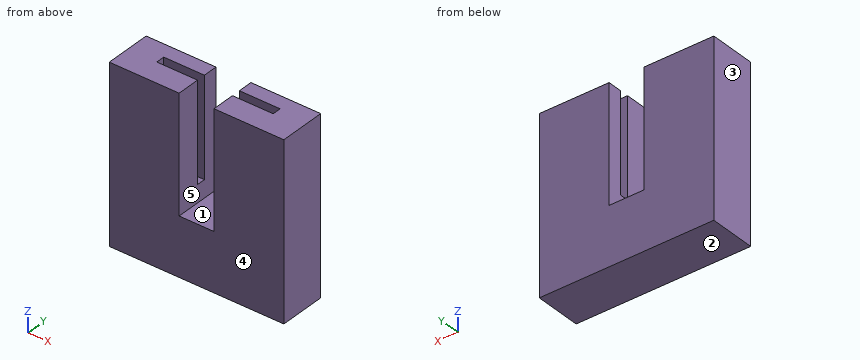
```python
from build123d import *

# Parameters (mm, degrees)
F0_W     = 30
F0_H     = 8
F1_DEPTH = 30
F3_W     = 6
F3_H     = 2.5
F3_H_2   = 4
F4_DEPTH = 20
F2_W     = 20
F2_H     = 1.5
F5_DEPTH = 20
F6_W     = 7
F6_H     = 1.5
F7_DEPTH = 3


with BuildPart() as f1:
    # F0 (on Top) → F1 (new body)
    with BuildSketch(Plane.XY):
        with Locations((-15, -4)):
            Rectangle(F0_W, F0_H)
    extrude(amount=F1_DEPTH)

    # F3 (on face) → F4 (cut)
    with BuildSketch(Plane.XY.offset(30)):
        with Locations((-15, -1.25)):
            Rectangle(F3_W, F3_H)
        with Locations((-15, -6)):
            Rectangle(F3_W, F3_H_2)
    extrude(amount=-F4_DEPTH, mode=Mode.SUBTRACT)

    # F2 (on face) → F5 (cut)
    with BuildSketch(Plane.XY.offset(30)):
        with Locations((-15, -3.25)):
            Rectangle(F2_W, F2_H)
    extrude(amount=-F5_DEPTH, mode=Mode.SUBTRACT)

    # F6 (on face) → F7 (join)
    with BuildSketch(Plane.XY.offset(10)):
        with Locations((-8.5, -3.25)):
            Rectangle(F6_W, F6_H)
        with Locations((-21.5, -3.25)):
            Rectangle(F6_W, F6_H)
    extrude(amount=F7_DEPTH)


solid = f1.part
```
For this review, take the finished solid that the model builds, in its own axes (mm). Face numbers are marked on the shaded views. A direction names the side the tool comes from. Coordinates: 2 decimals unless noted, no trailing zeros. Loops run counter-clockwise (first coordinate to the right, second up) from the corner with the lowest first, then second, coordinate; pieces in that order, holes last.
1. Add section B-B, the plane y = -5.25. Give the boundary of the cut face in (x, z), then the cut area to 3 significant figures.
2. Add section D-D, the plane z = 23.5. Give the boundary of the cut face in (x, y), then the cut area to 3 significant figures.
3. For the marked faces 4 and 5, list the 3-axis set-ups (+Z, -Z, +X, -X, +Y, -Y) from which the entire face can be reached by the end or side of a thin tool; tool diameter is ignored.
4. Add section C-C, the plane x = -8.25. Give the boundary of the cut face in (y, z).
5. Add section A-A, the plane z = 12.5. Give the boundary of the cut face in (x, y).
6. Mouldability with a two-part tool opening along X and no side actions: class the marked faces 1, 2 and 3 as +X half, -X half, draft (parallel to the pull), parting line (faces both ways), or undercut.
7. Insertion check: P1, Ø3.5, axis at x = -7.5, z = 18, coming from the +Y side; P2, Ø3, axis at x = -14, y = -4, coming from the +Z side. Each pin has a flat end and moves straight along its axis. Give the tip position at first contact, or say it passes through.
8. For line 1 (X direction, y = -6, z = 15); line 2 (Y direction, x = -8, z = 26); line 3 (X direction, y = -3.25, z = 28.25), list the stretches that pass through material, from the lowest coordinate up.
Result:
1. outline: (-30, 0) - (0, 0) - (0, 30) - (-12, 30) - (-12, 10) - (-18, 10) - (-18, 30) - (-30, 30) - close
1. area: 780 mm2
2. outline: (-30, -8) - (-18, -8) - (-18, -4) - (-25, -4) - (-25, -2.5) - (-18, -2.5) - (-18, 0) - (-30, 0) - close; (-12, -8) - (0, -8) - (0, 0) - (-12, 0) - (-12, -2.5) - (-5, -2.5) - (-5, -4) - (-12, -4) - close
2. area: 171 mm2
3. face 4: +Z, -Z, +X, -X, -Y
3. face 5: +Z, +Y, -Y
4. outline: (-8, 0) - (0, 0) - (0, 30) - (-2.5, 30) - (-2.5, 13) - (-4, 13) - (-4, 30) - (-8, 30) - close
5. outline: (-30, -8) - (-18, -8) - (-18, 0) - (-30, 0) - close; (-12, -8) - (0, -8) - (0, 0) - (-12, 0) - close
6. face 1: undercut
6. face 2: draft
6. face 3: -X half
7. P1: stops at y = 0
7. P2: stops at z = 10
8. line 1: x = -30 to -18, -12 to 0
8. line 2: y = -8 to -4, -2.5 to 0
8. line 3: x = -30 to -25, -5 to 0
